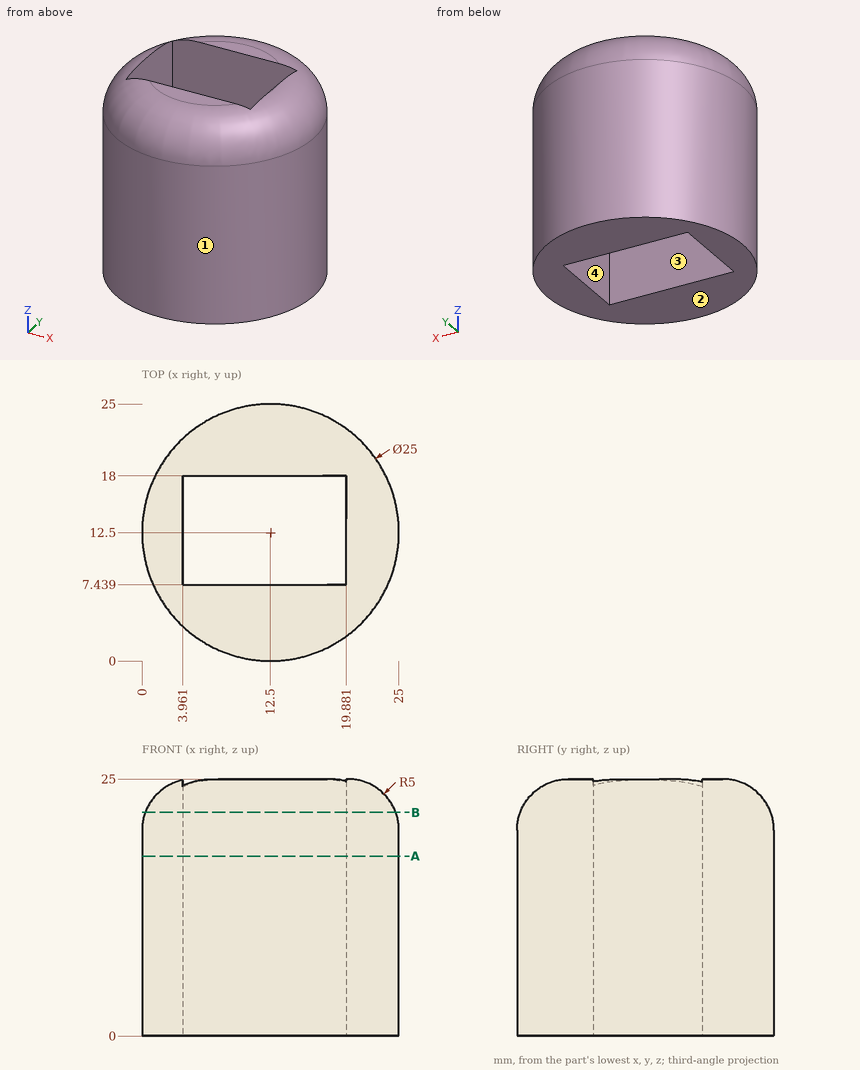
Input: dimensioned drawing with shaded views. Units: mm. Origin: part minimum x, y, z. Round coordinates to 2 decimals unless told otherwise and drop trailing zeros. Loops run counter-clockwise (first coordinate to the right, second up) from the corner with the lowest first, then second, coordinate; pieces in that order, holes last. Notation, with made-up numbers: (89, 85) -> (140, 85) arc R22 ccw to (140, 93) -> close; hole circle Ø5 at (67.25, 20.5). An arc over 180 degrees is marked (long way). Answer as a JSON object with one key per item and string values. Group by question number.
1) Pin query (flat end, axial travel): pin 1 (6 mm diameter, centred on x = 4, z = 13.5, fed in from -Y) (1 decimal); pin 2 (2 mm diameter, centred on y = 19.5, z = 21.5, fed in from -X); pin 3 (3 mm diameter, centred on y = 5, z = 12, fed in from -X). Return the tip coordinate at first contact, or that it passes through.
2) Section query A-A on z = 17.5. Output: boundary loops of the cut face in (x, y), plus the area to 3 significant figures.
3) Draft query along Y for the marked faces 1, 2, 3 and 4. Return one class per face: +Y half, -Y half, draft (parallel to the pull), parting line (faces both ways), or undercut.
4) Section query B-B on z = 21.75. Output: boundary loops of the cut face in (x, y).
5) Ray query, L1, parallel to X at y = 12.25, z = 12.5; L2, parallel to Y at x = 12.5, z = 10; L3, parallel to X at y = 16.25, z = 13.5 (1 decimal). Return the intervals inside material, ascending.
Reply:
{
 "1": {"pin 1": "stops at y = 1.3", "pin 2": "stops at x = 1.72", "pin 3": "stops at x = 1.53"},
 "2": {"outline": "circle Ø25 at (12.5, 12.5); hole (3.96, 7.44) -> (19.88, 7.44) -> (19.88, 18) -> (3.96, 18) -> close", "area": "323 mm2"},
 "3": {"face 1": "parting line", "face 2": "draft", "face 3": "undercut", "face 4": "undercut"},
 "4": {"outline": "circle Ø24.37 at (12.5, 12.5); hole (3.96, 7.44) -> (19.88, 7.44) -> (19.88, 18) -> (3.96, 18) -> close"},
 "5": {"L1": "x = 0 to 3.96, 19.88 to 25", "L2": "y = 0 to 7.44, 18 to 25", "L3": "x = 0.6 to 4, 19.9 to 24.4"}
}
